CAD build for the part. Positions are in the model's coordinates, mm. Face numbers are marked on the shaded views. Give positions to 0.01 mm unless a question says otherwise; leave off trailing zeros. Write each loop counter-clockwise with the first axis right and the second up, starting at its lowest first coordinate (ties: lowest second). Pieces come first, ordered by that corner, then holes. Notation, with made-up numbers: (63.5, 2.5) - (115.5, 2.5) arc R4 ccw to (115.5, 8.5) - close; hole circle Ø10 at (14, 75). An arc over 180 degrees is marked (long way). Answer as a JSON object with one key per item and string values.
from build123d import *

# Parameters (mm, degrees)
BOSS_EXTRUDE1_DEPTH = 4
BOSS_EXTRUDE2_DEPTH = 4


with BuildPart() as part:
    # Sketch1 → Boss-Extrude1 (new, symmetric)
    with BuildSketch(Plane(origin=(0, 0, 0), x_dir=(1, 0, 0), z_dir=(0, 0, -1))):
        with BuildLine():
            Line((-19, 9.5), (0, 9.5))
            ThreePointArc((0, 9.5), (5.676596321, 0), (0, -9.5))
            Line((0, -9.5), (-19, -9.5))
            ThreePointArc((-19, -9.5), (-8.500253603, -16.1800345), (3.912406176, -17.070771576))
            ThreePointArc((3.912406176, -17.070771576), (9.768875106, -14.366169937), (13.541125507, -9.133271576))
            ThreePointArc((13.541125507, -9.133271576), (15.24, 0), (13.541125507, 9.133271576))
            ThreePointArc((13.541125507, 9.133271576), (9.768875106, 14.366169937), (3.912406176, 17.070771576))
            ThreePointArc((3.912406176, 17.070771576), (-8.500253603, 16.1800345), (-19, 9.5))
        make_face()
    extrude(amount=BOSS_EXTRUDE1_DEPTH, both=True)

    # Sketch2 → Boss-Extrude2 (add, symmetric)
    with BuildSketch(Plane(origin=(0, 0, 0), x_dir=(1, 0, 0), z_dir=(0, 0, -1))):
        with BuildLine():
            Line((128.204707639, 10), (43.812088921, 10))
            ThreePointArc((43.812088921, 10), (30.504452796, 10.875291905), (17.426109311, 13.486086206))
            Line((17.426109311, 13.486086206), (4.988810205, 16.830875012))
            ThreePointArc((4.988810205, 16.830875012), (10.186731733, 14.006186237), (13.541125507, 9.133271576))
            ThreePointArc((13.541125507, 9.133271576), (15.24, 0), (13.541125507, -9.133271576))
            ThreePointArc((13.541125507, -9.133271576), (10.186731733, -14.006186237), (4.988810205, -16.830875012))
            Line((4.988810205, -16.830875012), (17.426109311, -13.486086206))
            ThreePointArc((17.426109311, -13.486086206), (30.504452796, -10.875291905), (43.812088921, -10))
            Line((43.812088921, -10), (128.204707639, -10))
            Line((128.204707639, -10), (150, -10))
            Line((150, -10), (150, 10))
            Line((150, 10), (128.204707639, 10))
        make_face()
    extrude(amount=BOSS_EXTRUDE2_DEPTH, both=True)


solid = part.part
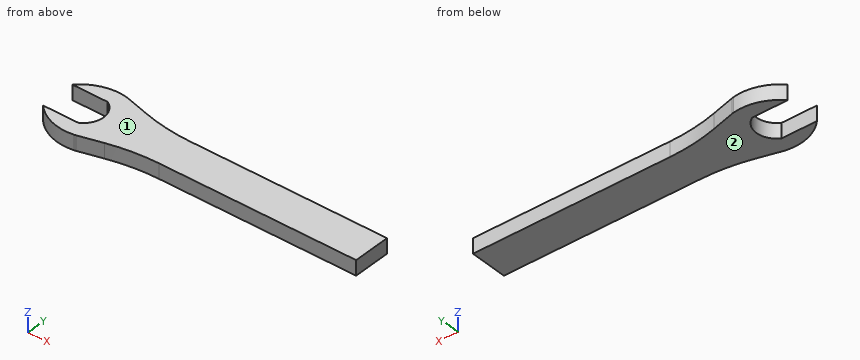
(1) Saw through at C-C, the plane x = 137.5. Give the cut face in (y, z).
Answer key:
{"outline": "(-10, -4) - (10, -4) - (10, 4) - (-10, 4) - close"}
(2) Flat gauge pins, fed straight in: P1, Ø1, axis at x = 120, z = -1, coming from the +Y side; P2, Ø2, axis at x = 64.5, z = 1, coming from the -Y side; P3, Ø1.5, axis at y = -6, z = 3, coming from the -X side; P4, Ø1, axis at x = 89, y = 11.5, coming from the +Z side. Where does each tip first touch, or does it go through?
Answer key:
{"P1": "stops at y = 10", "P2": "stops at y = -10", "P3": "stops at x = 3.3", "P4": "passes through"}
(3) Saw through at D-D, the plane y = 1.5. Give the cut face in (x, z).
Answer key:
{"outline": "(5.57, -4) - (150, -4) - (150, 4) - (5.57, 4) - close"}
(4) Saw through at A-A, the plane z = 0. Give the cut face in (x, y), and give its area (3 significant figures).
Answer key:
{"outline": "(-19, -9.5) arc R25.4 ccw to (3.91, -17.07) arc R12.7 ccw to (4.99, -16.83) - (17.43, -13.49) arc R101.6 cw to (43.81, -10) - (150, -10) - (150, 10) - (43.81, 10) arc R101.6 cw to (17.43, 13.49) - (4.99, 16.83) arc R12.7 ccw to (3.91, 17.07) arc R25.4 ccw to (-19, 9.5) - (0, 9.5) arc R10.79 cw to (0, -9.5) - close", "area": "3,400 mm²"}
(5) Saw through at B-B, the plane x = -4.5. Give the cut face in (y, z), and give its area (3 significant figures).
Answer key:
{"outline": "(-17.15, -4) - (-9.5, -4) - (-9.5, 4) - (-17.15, 4) - close; (9.5, -4) - (17.15, -4) - (17.15, 4) - (9.5, 4) - close", "area": "122 mm²"}
(6) Probe L1, parallel to Y at x = 48, z = -1.25; L2, parallel to Y at x = -1, z = 0.5; L3, parallel to Y at x = 2, z = 3.75. List the from-to ranges inside material, lowest first. Write a range as [from, to].
Answer key:
{"L1": "y = [-10, 10]", "L2": "y = [-17.46, -9.5], [9.5, 17.46]", "L3": "y = [-17.34, -8.11], [8.11, 17.34]"}
(7) Pull direction Z, two halves, no side cores. Call the marked faces 1 and 2: pulls with the +Z half, pulls with the -Z half, needs draft (parallel to the pull), parting line crosses it, or undercut.
Answer key:
{"face 1": "pulls with the +Z half", "face 2": "pulls with the -Z half"}
